from build123d import *

# Parameters (mm, degrees)
SKETCH_1_W      = 70
SKETCH_1_H      = 20
SKETCH_1_R      = 1.75
SKETCH_1_R_2    = 4.5
EXTRUDE_1_DEPTH = 4
SKETCH_1_3_W    = 5
SKETCH_1_3_H    = 20
EXTRUDE_2_DEPTH = 25


with BuildPart() as part:
    # Sketch 1 → Extrude 1 (new body)
    with BuildSketch(Plane(origin=(0, 0, 0), x_dir=(1, 0, 0), z_dir=(0, 1, 0))):
        with Locations((40, 10)):
            Rectangle(SKETCH_1_W, SKETCH_1_H)
        with Locations(Location((10, 10, 0), (0, 0, 270))):
            Circle(SKETCH_1_R, mode=Mode.SUBTRACT)
        with Locations(Location((23, 10, 0), (0, 0, 270))):
            Circle(SKETCH_1_R_2, mode=Mode.SUBTRACT)
        with Locations(Location((35, 10, 0), (0, 0, 270))):
            Circle(SKETCH_1_R, mode=Mode.SUBTRACT)
    extrude(amount=EXTRUDE_1_DEPTH)

    # Sketch 1_3 → Extrude 2 (add)
    with BuildSketch(Plane(origin=(0, 0, 0), x_dir=(1, 0, 0), z_dir=(0, 1, 0))):
        with Locations((2.5, 10)):
            Rectangle(SKETCH_1_3_W, SKETCH_1_3_H)
    extrude(amount=EXTRUDE_2_DEPTH)


solid = part.part
Design review of the part built by this model. Coordinates are the model's own, in mm. A direction names the side the tool comes from. Coordinates: 2 decimals unless noted, no trailing zeros. Loops run counter-clockwise (first coordinate to the right, second up) from the corner with the lowest first, then second, coordinate; pieces in that order, holes last.
Item 1: Add section A-A (x = 35). Write out the cut boundary in (y, z), and give its area (3 significant figures).
Completed:
outline: (0, -20) - (4, -20) - (4, -11.75) - (0, -11.75) - close; (0, -8.25) - (4, -8.25) - (4, 0) - (0, 0) - close
area: 66.0 mm2
Item 2: Draft analysis for pull direction X (two halves, no side actions). For faces 1 (the cylindrical face through (33.45, 1.97, -9.19)), 2 (the flat face through (26, 3, -20)), 3 (the flat face through (75, 2, -10)), state which applies: pulls with the +X half, pulls with the -X half, needs draft (parallel to the pull), parting line crosses it, or undercut.
Completed:
face 1: undercut
face 2: needs draft
face 3: pulls with the +X half
Item 3: For faces 4 (the flat face through (5, 14, -10)), 5 (the cylindrical face through (26.794, 1.972, -7.581)), list the 3-axis set-ups (+Z, -Z, +X, -X, +Y, -Y) from which the entire face can be reached by the end or side of a thin tool; tool diameter is ignored.
Completed:
face 4: +Z, -Z, +X, +Y
face 5: +Y, -Y
Item 4: Wall thickness on L1, parallel to X at y = 2.2, z = -10; L2, parallel to X at y = 10.5, z = -7.5; L3, parallel to Y at x = 18.5, z = -12: over which ranges is each line inside the solid? List them lowest first.
Completed:
L1: x = 0 to 8.25, 11.75 to 18.5, 27.5 to 33.25, 36.75 to 75
L2: x = 0 to 5
L3: y = 0 to 4
Item 5: Add section B-B (z = -10). Write out the cut boundary in (x, y).
Completed:
outline: (0, 0) - (8.25, 0) - (8.25, 4) - (5, 4) - (5, 25) - (0, 25) - close; (11.75, 0) - (18.5, 0) - (18.5, 4) - (11.75, 4) - close; (27.5, 0) - (33.25, 0) - (33.25, 4) - (27.5, 4) - close; (36.75, 0) - (75, 0) - (75, 4) - (36.75, 4) - close
Item 6: Clearance check with flat-ended pins moving along their axes: pin 1 (2 mm diameter, centred on x = 35, z = -10, fed in from +Y); pin 2 (6 mm diameter, centred on y = 16.5, z = -10, fed in from +X); pin 3 (1 mm diameter, centred on x = 28, z = -4, fed in from +Y); pin 4 (6 mm diameter, centred on y = 21.5, z = -6.5, fed in from -X). State where each tip first meets the part, or that it passes through.
Completed:
pin 1: passes through
pin 2: stops at x = 5
pin 3: stops at y = 4
pin 4: stops at x = 0
Item 7: Add section C-C (z = -2). Write out the cut boundary in (x, y), and give its area (3 significant figures).
Completed:
outline: (0, 0) - (75, 0) - (75, 4) - (5, 4) - (5, 25) - (0, 25) - close
area: 405 mm2
Item 8: Add section D-D (x = 23). Write out the cut boundary in (y, z).
Completed:
outline: (0, -20) - (4, -20) - (4, -14.5) - (0, -14.5) - close; (0, -5.5) - (4, -5.5) - (4, 0) - (0, 0) - close
